For this review, use the dimensioned drawing (mm, ordinates from the lowest corner) and the shaded views. Round coordinates to 2 decimals unless told otherwise and drop trailing zeros. Loops run counter-clockwise (first coordinate to the right, second up) from the corner with the lowest first, then second, coordinate; pieces in that order, holes last. Notation, with made-up numbers: M 4.25,45.5 L 30.25,45.5 A17 cw 30.25,61.5 Z; hole C 77.5,-23.5 d4. An arc over 180 degrees is marked long. One line per item, written item: value. Start each with the question number.
Item 1: We need section D-D (z = 35). Write out the cut boundary in (x, y).
Item 2: We need section B-B (x = 1). Write out the cut boundary in (y, z).
Item 3: For line 1 along Y through (x, z) = (0.7, 20); line 2 along Z through (x, y) = (1.75, 16); line 3 along Z through (x, y) = (1.65, 13.5) (1 decimal), list the stretches that pass through material, from the lowest coordinate up.
Item 4: We need section C-C (y = 19.5). Write out the cut boundary in (x, z).
Item 5: Clearance check with flat-ended pins moving along their axes: pin 1 (1 mm diameter, centred on x = 1.5, z = 22, fed in from +Y); pin 2 (1 mm diameter, centred on x = 1.5, z = 47, fed in from -Y) (3 decimals); pin 3 (1 mm diameter, centred on x = 0.5, y = 4, fed in from +Z). State where each tip first meets the part, or that it passes through.
Item 6: We need section A-A (z = 45). Write out the cut boundary in (x, y).
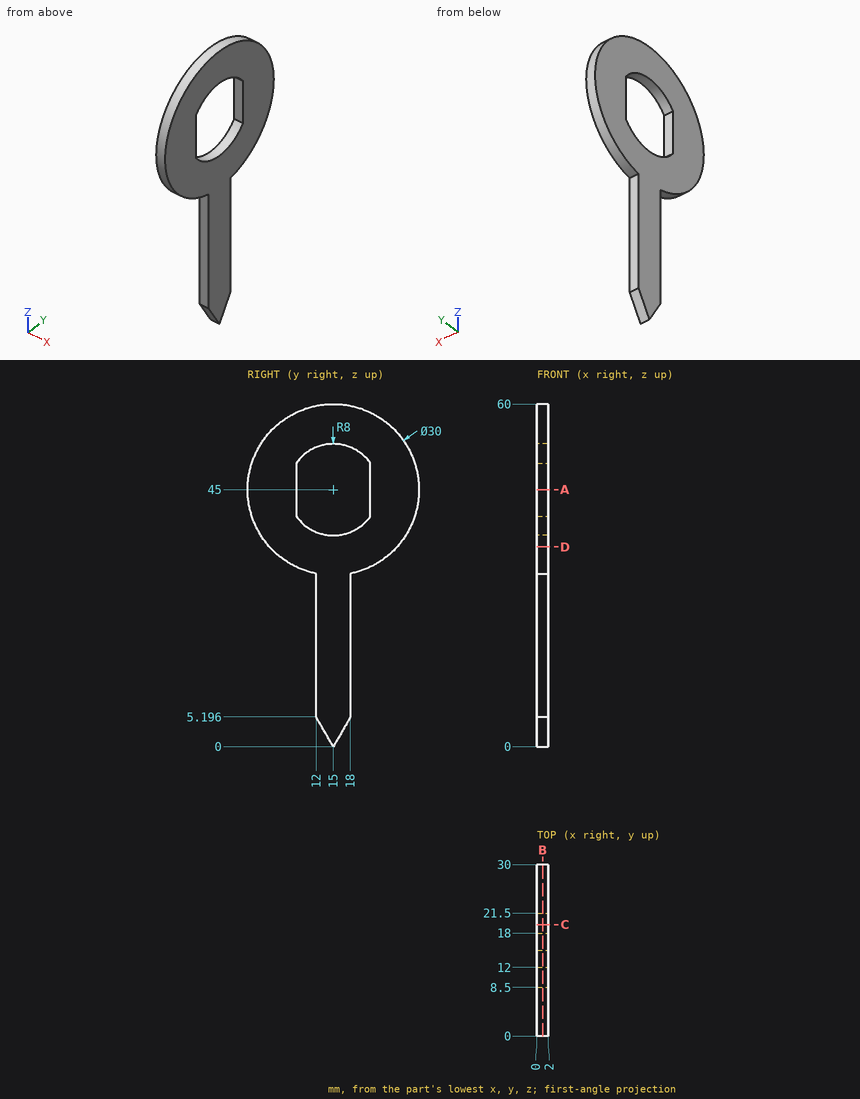
A:
1. outline: M 0,3.82 L 2,3.82 L 2,26.18 L 0,26.18 Z
2. outline: M 12,5.2 L 15,0 L 18,5.2 L 18,30.3 A15 ccw long 12,30.3 Z; hole M 8.5,40.34 A8 ccw 21.5,40.34 L 21.5,49.66 A8 ccw 8.5,49.66 Z
3. line 1: 12 to 18
3. line 2: 1.73 to 37.06, 52.94 to 59.97
3. line 3: 2.6 to 37.1, 52.9 to 59.9
4. outline: M 0,30.69 L 2,30.69 L 2,38.39 L 0,38.39 Z; M 0,51.61 L 2,51.61 L 2,59.31 L 0,59.31 Z
5. pin 1: y = 18
5. pin 2: y = 0.075
5. pin 3: z = 55.71
6. outline: M 0,0 L 2,0 L 2,8.5 L 0,8.5 Z; M 0,21.5 L 2,21.5 L 2,30 L 0,30 Z
